from build123d import *

# Parameters (mm, degrees)
SKETCH_1_W         = 108
SKETCH_1_H         = 61.7
PCB_DEPTH          = 1.6
SKETCH_2_W         = 95
SKETCH_2_H         = 61.2
EXTRUDE_560_DEPTH  = 4.5
SKETCH_4_W         = 3.5
SKETCH_4_H         = 36
EXTRUDE_3_DEPTH    = 1.5
EXTRUDE_START      = -1.6
SKETCH_4_2_W       = 3.5
SKETCH_4_2_H       = 36
EXTRUDE_4_DEPTH    = 8.5
HOLE_WIZARD_M3_1_D = 3.2


with BuildPart() as part:
    # 草图1 → PCB (new body)
    with BuildSketch(Plane(origin=(0, 0, 0), x_dir=(1, 0, 0), z_dir=(0, 1, 0))):
        Rectangle(SKETCH_1_W, SKETCH_1_H)
    extrude(amount=PCB_DEPTH)

    # 草图2 → Extrude 560 (add)
    with BuildSketch(Plane(origin=(0, 1.6, 0), x_dir=(1, 0, 0), z_dir=(0, 1, 0))):
        with Locations((0, -0.25)):
            Rectangle(SKETCH_2_W, SKETCH_2_H)
    extrude(amount=EXTRUDE_560_DEPTH)

    # 草图4 → 凸台-拉伸3 (add)
    with BuildSketch(Plane(origin=(0, 1.6, 0), x_dir=(1, 0, 0), z_dir=(0, 1, 0))):
        with Locations((-52.25, 0)):
            Rectangle(SKETCH_4_W, SKETCH_4_H)
    extrude(amount=EXTRUDE_3_DEPTH)

    # 草图4<2> → 凸台-拉伸4 (add)
    with BuildSketch(Plane(origin=(0, 1.6, 0), x_dir=(1, 0, 0), z_dir=(0, 1, 0)).offset(EXTRUDE_START)):
        with Locations((-52.25, 0)):
            Rectangle(SKETCH_4_2_W, SKETCH_4_2_H)
    extrude(amount=-EXTRUDE_4_DEPTH)

    # M3 间隙孔1 (through all)
    with Locations(Plane(origin=(0, 1.6, 0), x_dir=(1, 0, 0), z_dir=(0, 1, 0))):
        with Locations((-51, 27.5), (-51, -27.5), (51, 27.5), (51, -27.5)):
            Hole(HOLE_WIZARD_M3_1_D / 2)


solid = part.part
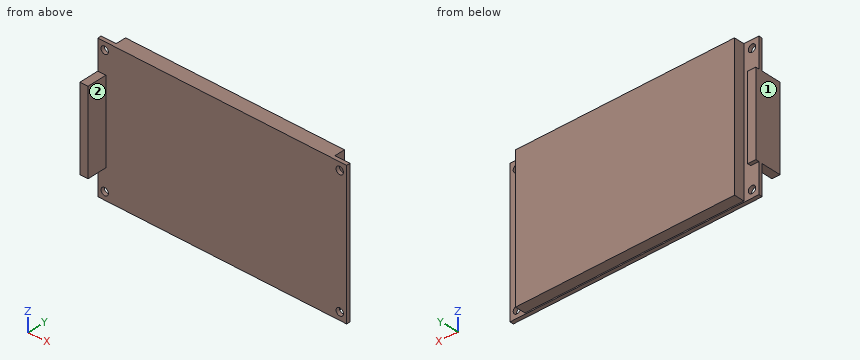
The model under review builds one solid part; all positions refer to its coordinate system, in mm. Face numbers are marked on the shaded views. A direction names the side the tool comes from. Round coordinates to 2 decimals unless told otherwise and drop trailing zeros. Loops run counter-clockwise (first coordinate to the right, second up) from the corner with the lowest first, then second, coordinate; pieces in that order, holes last. Notation, with made-up numbers: (42, 19.5) - (56, 19.5) arc R14 cw to (56, 32.5) - close; hole circle Ø11 at (59, -30). An arc over 180 degrees is marked (long way). Use CSV: the item, a comma, the result in double quotes.
(1) Clearance check with flat-ended pins moving along their axes: P1, Ø8, axis at x = 41.5, z = 23, coming from the -Y side; P2, Ø1.8, axis at x = -53, y = -2.5, coming from the +Z side; P3, Ø3, axis at x = -52, y = -5, coming from the -Z side; P4, Ø2, axis at y = -0.5, z = 21.5, coming from the +X side. State where each tip first meets the part, or that it passes through.
Working result:
P1,"stops at y = 0"
P2,"stops at z = 18"
P3,"stops at z = -18"
P4,"stops at x = 54"
(2) Machinability: for the marked faces 1 and 2, which of the approach directions +Z, -Z, +X, -X, +Y, -Y give a long, thin tool a straight path to every point of the face, cutting with its end or side? Answer none if there is none.
Working result:
face 1,"+Z, -Z, -X, +Y, -Y"
face 2,"+Z, -Z, +X, -Y"
(3) Take a section at D-D, the plane z = 15. Give the boundary of the cut face in (x, y), plus the area to 3 significant figures.
Working result:
outline,"(-54, -8.5) - (-50.5, -8.5) - (-50.5, 0) - (54, 0) - (54, 1.6) - (47.5, 1.6) - (47.5, 6.1) - (-47.5, 6.1) - (-47.5, 1.6) - (-50.5, 1.6) - (-50.5, 3.1) - (-54, 3.1) - close"
area,"635 mm^2"
(4) For line 1 (X direction, y = 0.75, z = -27.5); line 2 (Z direction, x = -51, y = 0.55); line 3 (X direction, y = 2.25, z = 3.5), list the stretches that pass through material, from the lowest coordinate up.
Working result:
line 1,"x = -54 to -52.6, -49.4 to 49.4, 52.6 to 54"
line 2,"z = -30.85 to -29.1, -25.9 to 25.9, 29.1 to 30.85"
line 3,"x = -54 to -50.5, -47.5 to 47.5"
(5) Take a section at B-B, the plane z = -27.5. Give the boundary of the cut face in (x, y).
Working result:
outline,"(-54, 0) - (-52.6, 0) - (-52.6, 1.6) - (-54, 1.6) - close; (-49.4, 0) - (49.4, 0) - (49.4, 1.6) - (47.5, 1.6) - (47.5, 6.1) - (-47.5, 6.1) - (-47.5, 1.6) - (-49.4, 1.6) - close; (52.6, 0) - (54, 0) - (54, 1.6) - (52.6, 1.6) - close"
(6) Take a section at A-A, the plane x = 51. Give the boundary of the cut face in (y, z), plus the area to 3 significant figures.
Working result:
outline,"(0, -30.85) - (1.6, -30.85) - (1.6, -29.1) - (0, -29.1) - close; (0, -25.9) - (1.6, -25.9) - (1.6, 25.9) - (0, 25.9) - close; (0, 29.1) - (1.6, 29.1) - (1.6, 30.85) - (0, 30.85) - close"
area,"88.5 mm^2"
(7) Take a section at C-C, the plane x = -44.5. Give the boundary of the cut face in (y, z).
Working result:
outline,"(0, -30.85) - (1.6, -30.85) - (1.6, -30.35) - (6.1, -30.35) - (6.1, 30.85) - (0, 30.85) - close"
